Autodesk Inventor part; units mm, degrees
ref_plane "YZ Plane" through (0, 0, 0) normal (1, 0, 0) x (0, 1, 0)
ref_plane "XZ Plane" through (0, 0, 0) normal (0, 1, 0) x (-1, 0, 0)
ref_plane "XY Plane" through (0, 0, 0) normal (0, 0, 1) x (1, 0, 0)
sketch "Sketch1" plane through (0, 0, 0) normal (0, 1, 0) x (-1, 0, 0)
  line L0 (24, 138) -> (-24, 138)
  line L1 (-24, 138) -> (-24, -138)
  line L2 (-24, -138) -> (24, -138)
  line L3 (24, -138) -> (24, 138)
  point P0 (0, 0)
  dimension "d0" = 48
  dimension "d1" = 276
extrude "Extrusion1" add sketch "Sketch1" along normal blind 3
sketch "Sketch2" plane through (0, 3, 0) normal (0, 1, 0) x (1, 0, 0)
  line L0 (-24, 138) -> (-24, -138)
  line L1 (-24, -138) -> (-20, -138)
  line L2 (-20, -138) -> (-20, -90)
  line L3 (-20, -90) -> (-24, -90)
  line L4 (-24, -90) -> (-24, -138)
  line L5 (24, -138) -> (24, 138)
  line L6 (-20, -90) -> (24, -90)
  line L7 (24, -90) -> (24, -94)
  line L8 (24, -94) -> (-20, -94)
  line L9 (-20, -94) -> (-20, -90)
  line L10 (-24, -138) -> (24, -138)
  line L11 (24, -94) -> (20, -94)
  line L12 (20, -94) -> (20, -138)
  line L13 (20, -138) -> (24, -138)
  line L14 (24, -138) -> (24, -94)
  line L15 (20, -138) -> (-20, -138)
  line L16 (-20, -138) -> (-20, -134)
  line L17 (-20, -134) -> (20, -134)
  line L18 (20, -134) -> (20, -138)
  point P0 (0, 0)
  dimension "d4" = 4
  dimension "d5" = 48
  dimension "d6" = 4
  dimension "d7" = 4
  dimension "d8" = 4
extrude "Extrusion2" add sketch "Sketch2" along normal blind 3 contours L3 L2 L1 L0 | L6 L5 L8 L2 | L2 L17 L12 L10 | L12 L8 L5 L10
mirror "Mirror1" about plane through (0, 0, 0) normal (0, 0, 1) of "Extrusion2"
sketch "Sketch3" plane through (0, 0, 0) normal (0, -1, 0) x (1, 0, 0)
  line L0 (24, -90) -> (-24, -90)
  line L1 (24, 138) -> (24, -138)
  line L2 (-24, -90) -> (24, -90)
  line L3 (24, -90) -> (24, -93)
  line L4 (24, -93) -> (-24, -93)
  line L5 (-24, -93) -> (-24, -90)
  line L6 (-24, 90) -> (24, 90)
  line L7 (24, 90) -> (21, 90)
  line L8 (21, 90) -> (21, -90)
  line L9 (21, -90) -> (24, -90)
  line L10 (24, -90) -> (24, 90)
  line L11 (-24, 90) -> (24, 90)
  line L12 (24, 90) -> (24, 93)
  line L13 (24, 93) -> (-24, 93)
  line L14 (-24, 93) -> (-24, 90)
  point P0 (0, 0)
  dimension "d11" = 3
  dimension "d12" = 3
  dimension "d13" = 3
extrude "Extrusion3" add sketch "Sketch3" along normal blind 35
sketch "Sketch4" plane through (-24, 0, -90) normal (0, 0, 1) x (1, 0, 0)
  line L0 (0, -35) -> (45, -35)
  line L1 (45, 0) -> (45, -35)
  line L2 (0, -35) -> (45, -35)
  line L3 (45, -35) -> (45, -31)
  line L4 (45, -31) -> (0, -31)
  line L5 (0, -31) -> (0, -35)
  point P0 (24, 0)
  dimension "d16" = 4
extrude "Extrusion4" add sketch "Sketch4" along normal blind 8
sketch "Sketch5" plane through (-24, -31, -90) normal (0, 1, 0) x (1, 0, 0)
  line L0 (0, -8) -> (45, -8)
  line L1 (45, 0) -> (45, -8)
  line L2 (0, -8) -> (45, -8)
  line L3 (45, -8) -> (45, -4)
  line L4 (45, -4) -> (0, -4)
  line L5 (0, -4) -> (0, -8)
  point P0 (24, -90)
  dimension "d19" = 4
extrude "Extrusion5" add sketch "Sketch5" along normal blind 4
sketch "Sketch6" plane through (0, 0, 0) normal (0, -1, 0) x (1, 0, 0)
  line L0 (21, -86) -> (-24, -86)
  line L1 (-24, -82) -> (21, -82)
  line L2 (21, -82) -> (21, -86)
  line L3 (21, -86) -> (-24, -86)
  line L4 (-24, -86) -> (-24, -82)
  point P0 (0, 0)
  dimension "d22" = 4
extrude "Extrusion6" add sketch "Sketch6" along normal blind 4
mirror "Mirror2" about plane through (0, 0, 0) normal (0, 0, 1) of "Extrusion6", "Extrusion5", "Extrusion4"
sketch "Sketch7" plane through (0, 0, 0) normal (0, -1, 0) x (1, 0, 0)
  circle A0 centre (-14, -127) radius 3
  circle A1 centre (14, -127) radius 3
  circle A2 centre (14, -101) radius 3
  circle A3 centre (-14, -101) radius 3
  line L0 (-20, -94) -> (20, -94)
  line L1 (20, -134) -> (-20, -134)
  line L2 (20, -94) -> (20, -134)
  point P0 (0, 0)
  dimension "d25" = 6
  dimension "d26" = 6
  dimension "d27" = 6
  dimension "d28" = 6
  dimension "d80" = 28
  dimension "d81" = 26
  dimension "d82" = 26
  dimension "d83" = 28
  dimension "d84" = 7
  dimension "d85" = 7
  dimension "d86" = 7
  dimension "d87" = 6
extrude "Extrusion7" cut sketch "Sketch7" against normal blind 4
mirror "Mirror3" about plane through (0, 0, 0) normal (0, 0, 1) of "Extrusion7"
sketch "Sketch12" plane through (0, 0, 0) normal (0, -1, 0) x (1, 0, 0)
  line L0 (-24, -82) -> (-24, 82)
  line L1 (-24, 0) -> (24, 0)
  line L2 (24, 0) -> (24, 138)
  line L3 (24, 138) -> (-24, 138)
  line L4 (-24, 138) -> (-24, 0)
  point P0 (0, 0)
  point P1 (-24, -17)
extrude "Extrusion12" cut sketch "Sketch12" along normal mid plane 100
sketch "Sketch13" plane through (0, 0, 0) normal (0, -1, 0) x (1, 0, 0)
  line L0 (-24, -90) -> (-24, 0)
  line L1 (-24, -10) -> (-9, -10)
  line L2 (-9, -10) -> (-9, 10)
  line L3 (-9, 10) -> (-24, 10)
  line L4 (-24, 10) -> (-24, -10)
  line L5 (6, -10) -> (21, -10)
  line L6 (21, -10) -> (21, 10)
  line L7 (21, 10) -> (6, 10)
  line L8 (6, 10) -> (6, -10)
  point P0 (0, 0)
  dimension "d55" = 15
  dimension "d56" = 20
  dimension "d57" = 15
  dimension "d58" = 20
extrude "Extrusion13" add sketch "Sketch13" along normal blind 4 and the other way blind 7
sketch "Sketch14" plane through (21, -31, -90) normal (-1, 0, 0) x (0, 0, 1)
  point P0 (90, 31)
sketch "Sketch15" plane through (21, -31, -90) normal (-1, 0, 0) x (0, 0, 1)
  line L0 (90, -4) -> (8, -4)
  line L1 (80, -4) -> (100, -4)
  line L2 (100, -4) -> (100, 11)
  line L3 (100, 11) -> (80, 11)
  line L4 (80, 11) -> (80, -4)
  point P0 (90, 31)
  dimension "d63" = 20
  dimension "d64" = 15
extrude "Extrusion14" add sketch "Sketch15" along normal blind 4 and the other way blind 7
sketch "Sketch16" plane through (0, -4, 0) normal (0, -1, 0) x (1, 0, 0)
  circle A0 centre (-16.5, 5) radius 2
  circle A1 centre (13.5, 5) radius 2
  circle A2 centre (-1.5, -5) radius 2
  point P0 (0, 0)
  dimension "d69" = 4
  dimension "d70" = 4
  dimension "d71" = 4
extrude "Extrusion15" cut sketch "Sketch16" against normal blind 20
sketch "Sketch17" plane through (17, -31, -90) normal (-1, 0, 0) x (0, 0, 1)
  circle A0 centre (95, 3.5) radius 2
  circle A1 centre (85, 18.5) radius 2
  point P0 (90, 31)
  dimension "d74" = 4
  dimension "d75" = 4
extrude "Extrusion16" cut sketch "Sketch17" against normal blind 20
sketch "Sketch18" plane through (-24, -4, 10) normal (0, 0, 1) x (1, 0, 0)
  line L0 (48, 4) -> (48, -31)
  line L1 (45, -31) -> (45, -16)
  line L2 (48, -31) -> (45, -31)
  line L3 (45, -31) -> (45, -16)
  line L4 (45, -16) -> (48, -16)
  line L5 (48, -16) -> (48, -31)
  line L6 (48, 7) -> (0, 7)
  line L7 (45, 4) -> (0, 4)
  line L8 (0, 4) -> (0, 7)
  line L9 (0, 7) -> (45, 7)
  line L10 (45, 7) -> (45, 4)
  point P0 (24, 4)
extrude "Extrusion17" cut sketch "Sketch18" against normal blind 10
fillet "Fillet1" radius 2 7 edges at (24, -35, -51.5) (24, 3, -45) (-24, 3, -50) (-24, 0, -115.5) (0, 0, -138) (24, 0, -115.5) (0, -35, -93)
properties part number "carriageEnd2R"
Input: part model. Units: mm. Frame: model coordinates. A direction names the side the tool comes from. Coordinates: 2 decimals unless noted, no trailing zeros. Loops run counter-clockwise (first coordinate to the right, second up) from the corner with the lowest first, then second, coordinate; pieces in that order, holes last. Notation, with made-up numbers: (28, 11) -> (32, 11) arc R19 cw to (32, 31) -> close; hole circle Ø2 at (31, -9.5). An arc over 180 degrees is marked (long way). Write item = value, one per line. Start each with the question number.
Item 1: Cut plane B-B, the plane y = -12.5. Return loops of the section in (x, z), plus the area to 3 significant figures.
Item 2: Mould query, pull axis X, two halves, no side actions, for faces 1 (the face through (-9, -2, 0)), 2 (the face through (-24, -3.2, -85.6)), 3 (the face through (-2, -31, -82)). Classes: pulls with the +X half, pulls with the -X half, needs draft (parallel to the pull), parting line crosses it, or undercut.
Item 3: Reachability of faces 4 (the face through (-1, 0, -88)), 5 (the face through (21, 5, 0)), 6 (the face through (15.3, 3, 6.2)) from +Z, -Z, +X, -X, +Y, -Y: full face, straight path, thin tool, end or side. Return the list, or none.
Item 4: Cut plane C-C, the plane x = -6. Return loops of the section in (y, z), plus the area to 3 significant figures.
Item 5: Cut plane A-A, the plane z = -127. Return loops of the section in (x, y), plus the area to 3 significant figures.
Item 6: First-contact query: P1, Ø1.5, axis at x = -4.5, y = -0.5, coming from the -Z side; P2, Ø1.2, axis at y = 6, z = -1, coming from the +X side; P3, Ø24, axis at x = -11.5, z = -111.5, coming from the +Y side. Flat tips, straight axial feed; report the tip coordinate or a pass-through.
Item 7: Material intervals for line 1 (Z direction, x = -16.5, y = 5.05); line 2 (Y direction, x = 19, z = -0.5); line 3 (Z direction, x = -14, y = 1.2), sorted ascending.
Item 8: Cut plane D-D, the plane z = -12. Return loops of the section in (x, y).
Ans:
q1.outline = (-24, -93) -> (24, -93) -> (24, -7) -> (21, -7) -> (21, -90) -> (-24, -90) -> close; (21, -3) -> (24, -3) -> (24, 0) -> (21, 0) -> close
q1.area = 402 mm²
q2.face_1 = undercut
q2.face_2 = pulls with the -X half
q2.face_3 = needs draft
q3.face_4 = -X
q3.face_5 = +Z, +X, +Y
q3.face_6 = +Z, +X, -X
q4.outline = (-35, -91) arc R2 ccw to (-33, -93) -> (0, -93) -> (0, -136) arc R2 ccw to (2, -138) -> (6, -138) -> (6, -134) -> (3, -134) -> (3, -94) -> (6, -94) -> (6, -90) -> (3, -90) -> (3, 0) -> (0, 0) -> (0, -82) -> (-4, -82) -> (-4, -86) -> (0, -86) -> (0, -90) -> (-31, -90) -> (-31, -86) -> (-27, -86) -> (-27, -82) -> (-35, -82) -> close
q4.area = 605 mm²
q5.outline = (-24, 2) arc R2 ccw to (-22, 0) -> (-17, 0) -> (-17, 3) -> (-20, 3) -> (-20, 6) -> (-24, 6) -> close; (-11, 0) -> (11, 0) -> (11, 3) -> (-11, 3) -> close; (17, 0) -> (22, 0) arc R2 ccw to (24, 2) -> (24, 6) -> (20, 6) -> (20, 3) -> (17, 3) -> close
q5.area = 130 mm²
q6.P1 = -136.97
q6.P2 = 21
q6.P3 = 6
q7.line_1 = -138 to -134, -94 to -90, -10 to 3, 7 to 10
q7.line_2 = -35 to -20, -4 to 7
q7.line_3 = -137.83 to -130, -124 to -104, -98 to 0
q8.outline = (-24, 0) -> (21, 0) -> (21, -35) -> (22, -35) arc R2 ccw to (24, -33) -> (24, 1) arc R2 ccw to (22, 3) -> (-22, 3) arc R2 ccw to (-24, 1) -> close
